For this review, use the dimensioned drawing (mm, ordinates from the lowest corner) and the shaded views. A direction names the side the tool comes from. Round coordinates to 2 decimals unless told otherwise and drop trailing zeros. Order: outer loops, then holes, each group sorted by start corner. A loop starts at its lowest first (then second) coordinate and runs counter-clockwise, first axis right, second up. Notation, with made-up numbers: M 49.25,17 L 87.25,17 A23 ccw 87.25,27 Z; hole C -2.75,38.5 d8. An arc over 180 degrees is marked long. Use a Markdown table: item, result. Add a question column.
1. The part is to be moulded in two halves that separate along Z. For the marked faces 3, 4, 5 and 6, say which applies: +Z half, -Z half, draft (parallel to the pull), parting line (faces both ways), or undercut.
2. Consider section C-C on y = 7.5. State the section outline as (x, z) points.
3. For the marked faces 1 and 2, list the 3-axis set-ups (+Z, -Z, +X, -X, +Y, -Y) from which the entire face can be reached by the end or side of a thin tool; tool diameter is ignored.
4. To check wall thickness, follow probe 1 along X at (y, z) = (15.5, 7.25); probe 2 along X at (y, z) = (7.5, 0.25). State the ranges of each line that lie inside material, in increasing order.
5. Consider section D-D on x = 4.5. State the section outline as (y, z) points.
6. Consider section A-A on x = 2.25. State the section outline as (y, z) points.
7. Consider section B-B on z = 7.25. State the section outline as (x, y) points.
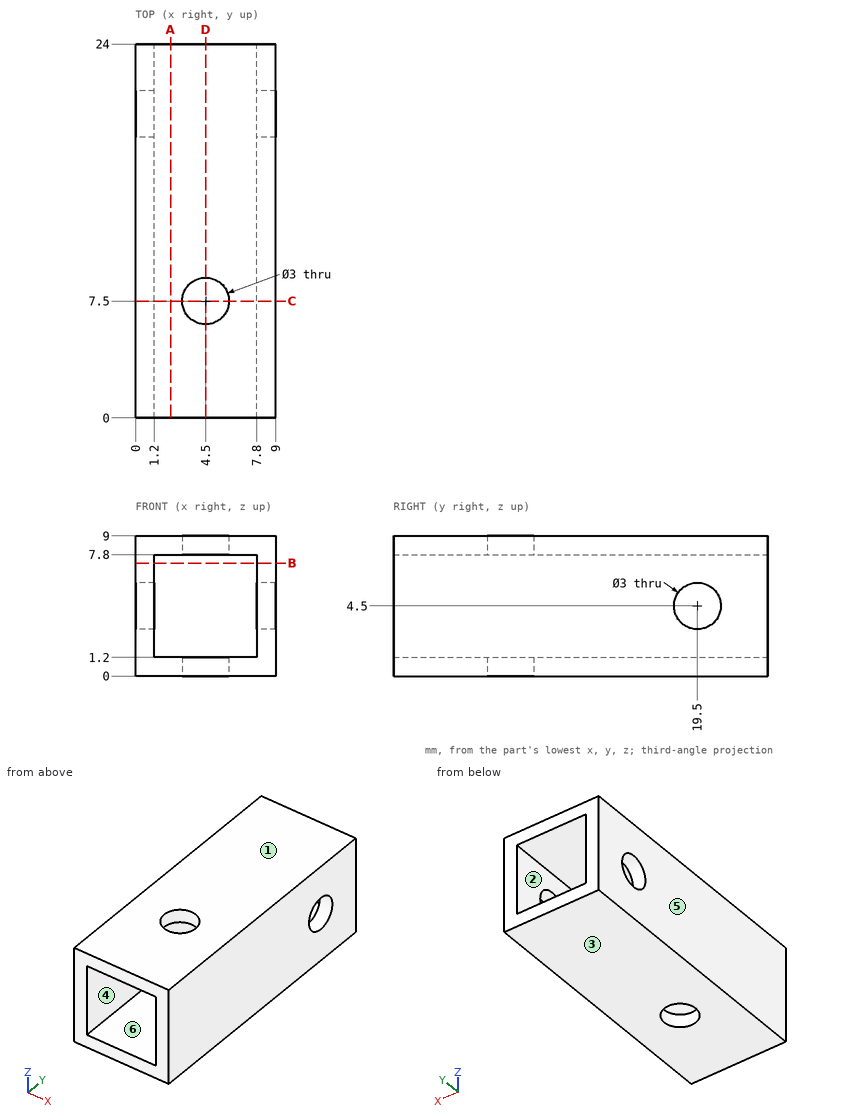
Answer block:
| question | item | result |
|---|---|---|
| 1 | face 3 | -Z half |
| 1 | face 4 | undercut |
| 1 | face 5 | draft |
| 1 | face 6 | undercut |
| 2 | outline | M 0,0 L 3,0 L 3,1.2 L 1.2,1.2 L 1.2,7.8 L 3,7.8 L 3,9 L 0,9 Z; M 6,0 L 9,0 L 9,9 L 6,9 L 6,7.8 L 7.8,7.8 L 7.8,1.2 L 6,1.2 Z |
| 3 | face 1 | +Z, +X, -X, +Y, -Y |
| 3 | face 2 | +Y, -Y |
| 4 | probe 1 | 0 to 1.2, 7.8 to 9 |
| 4 | probe 2 | 0 to 3, 6 to 9 |
| 5 | outline | M 0,0 L 6,0 L 6,1.2 L 0,1.2 Z; M 0,7.8 L 6,7.8 L 6,9 L 0,9 Z; M 9,0 L 24,0 L 24,1.2 L 9,1.2 Z; M 9,7.8 L 24,7.8 L 24,9 L 9,9 Z |
| 6 | outline | M 0,0 L 24,0 L 24,1.2 L 0,1.2 Z; M 0,7.8 L 24,7.8 L 24,9 L 0,9 Z |
| 7 | outline | M 0,0 L 1.2,0 L 1.2,24 L 0,24 Z; M 7.8,0 L 9,0 L 9,24 L 7.8,24 Z |
